```python
from build123d import *

# Parameters (mm, degrees)
SKETCH_1_W          = 75
SKETCH_1_H          = 273
EXTRUDE_1_DEPTH     = 25
SKETCH_2_R          = 10.5
CUT_EXTRUDE_1_DEPTH = 26
CHAMFER_1_SIZE      = 6
CHAMFER_1_SIZE2     = 10.392304845
CHAMFER_2_SIZE      = 6
CHAMFER_2_SIZE2     = 10.392304845


with BuildPart() as part:
    # Эскиз1 → Бобышка-Вытянуть1 (new body)
    with BuildSketch(Plane.XY):
        with Locations((37.5, 136.5)):
            Rectangle(SKETCH_1_W, SKETCH_1_H)
    extrude(amount=EXTRUDE_1_DEPTH)

    # Эскиз2 → Вырез-Вытянуть1 (cut, through all)
    with BuildSketch(Plane.XY.offset(25)):
        with Locations((37.5, 23)):
            Circle(SKETCH_2_R)
        with Locations((37.5, 73)):
            Circle(SKETCH_2_R)
        with Locations((37.5, 123)):
            Circle(SKETCH_2_R)
        with Locations((37.5, 173)):
            Circle(SKETCH_2_R)
        with Locations((37.5, 223)):
            Circle(SKETCH_2_R)
    extrude(amount=-CUT_EXTRUDE_1_DEPTH, mode=Mode.SUBTRACT)

    # Фаска1
    chamfer_1_edges = [part.edges().sort_by_distance(p)[0] for p in [
        (37.5, 0, 0),
    ]]
    chamfer_1_side = [part.faces().sort_by_distance(p)[0] for p in [
        (37.5, 137.747350693, 0),
    ]]
    chamfer(chamfer_1_edges, length=CHAMFER_1_SIZE, length2=CHAMFER_1_SIZE2, reference=chamfer_1_side[0])

    # Фаска2
    chamfer_2_edges = [part.edges().sort_by_distance(p)[0] for p in [
        (37.5, 0, 25),
    ]]
    chamfer_2_side = [part.faces().sort_by_distance(p)[0] for p in [
        (37.5, 137.747350693, 25),
    ]]
    chamfer(chamfer_2_edges, length=CHAMFER_2_SIZE, length2=CHAMFER_2_SIZE2, reference=chamfer_2_side[0])


solid = part.part
```
Work out the finished part from the listing and answer in its coordinate system (mm). Round coordinates to 2 decimals unless told otherwise and drop trailing zeros. Write each loop counter-clockwise with the first axis right and the second up, starting at its lowest first coordinate (ties: lowest second). Pieces come first, ordered by that corner, then holes.
1) Consider probe 1 along Y at (x, z) = (37.5, 12.25); probe 2 along Y at (x, z) = (40, 14.25); probe 3 along Y at (x, z) = (52.5, 5.25). Determine where each line is inside the solid, lowest interval first.
2) A cutting plane is placed at A-A on y = 123. Determine the outline of the cut face in (x, z), and give its area (3 significant figures).
3) A cutting plane is placed at C-C on x = 41.5. Determine the outline of the cut face in (y, z), and give its area (3 significant figures).
4) Determine the mould class of faces 1 (the face through (27, 23, 13)), 2 (the face through (0, 135, 12)), 3 (the face through (36.975, 2.958, 5.269)) for opening direction X: pulls with the +X half, pulls with the -X half, needs draft (parallel to the pull), parting line crosses it, or undercut.
5) A cutting plane is placed at B-B on z = 7.25. Determine the outline of the cut face in (x, y).
6) A cutting plane is placed at D-D on z = 21.5. Determine the outline of the cut face in (x, y).
Entries:
1. probe 1: y = 0 to 12.5, 33.5 to 62.5, 83.5 to 112.5, 133.5 to 162.5, 183.5 to 212.5, 233.5 to 273
1. probe 2: y = 0 to 12.8, 33.2 to 62.8, 83.2 to 112.8, 133.2 to 162.8, 183.2 to 212.8, 233.2 to 273
1. probe 3: y = 2.97 to 273
2. outline: (0, 0) - (27, 0) - (27, 25) - (0, 25) - close; (48, 0) - (75, 0) - (75, 25) - (48, 25) - close
2. area: 1,350 mm2
3. outline: (0, 10.39) - (6, 0) - (13.29, 0) - (13.29, 25) - (6, 25) - (0, 14.61) - close; (32.71, 0) - (63.29, 0) - (63.29, 25) - (32.71, 25) - close; (82.71, 0) - (113.29, 0) - (113.29, 25) - (82.71, 25) - close; (132.71, 0) - (163.29, 0) - (163.29, 25) - (132.71, 25) - close; (182.71, 0) - (213.29, 0) - (213.29, 25) - (182.71, 25) - close; (232.71, 0) - (273, 0) - (273, 25) - (232.71, 25) - close
3. area: 4,340 mm2
4. face 1: undercut
4. face 2: pulls with the -X half
4. face 3: needs draft
5. outline: (0, 1.81) - (75, 1.81) - (75, 273) - (0, 273) - close; hole circle Ø21 at (37.5, 23); hole circle Ø21 at (37.5, 73); hole circle Ø21 at (37.5, 123); hole circle Ø21 at (37.5, 173); hole circle Ø21 at (37.5, 223)
6. outline: (0, 3.98) - (75, 3.98) - (75, 273) - (0, 273) - close; hole circle Ø21 at (37.5, 23); hole circle Ø21 at (37.5, 73); hole circle Ø21 at (37.5, 123); hole circle Ø21 at (37.5, 173); hole circle Ø21 at (37.5, 223)
